```python
from build123d import *

# Parameters (mm, degrees)
F0_W     = 1168.9519882202
F0_H     = 1194.2882537842
F1_DEPTH = 152.4
F2_T     = 25.4


with BuildPart() as f1:
    # F0 (on Top) → F1 (new body)
    with BuildSketch(Plane.XY):
        Rectangle(F0_W, F0_H)
    extrude(amount=F1_DEPTH)

    # F2
    f2_openings = [f1.faces().sort_by_distance(p)[0] for p in [
        (0, 0, 0),
        (0, 0, 152.4),
    ]]
    offset(amount=F2_T, openings=f2_openings, kind=Kind.INTERSECTION)


solid = f1.part
```
CAD build for the part. Positions are in the model's coordinates, mm. A direction names the side the tool comes from. Give positions to 0.01 mm unless a question says otherwise; leave off trailing zeros. Loops run counter-clockwise (first coordinate to the right, second up) from the corner with the lowest first, then second, coordinate; pieces in that order, holes last. Notation, with made-up numbers: (-13.5, 76) -> (28.5, 76) arc R27 cw to (28.5, 101) -> close; hole circle Ø3 at (20, 35). An arc over 180 degrees is marked (long way). Use a Markdown table: item, result.
1. Mould opens along Y. For faces 1 (the flat face through (-8, -597.144, 75)), 2 (the flat face through (-590, 280, 152.4)), 3 (the flat face through (-584.476, -8, 75)), 4 (the flat face through (-9, 622.544, 75)) say: pulls with the +Y half, pulls with the -Y half, needs draft (parallel to the pull), parting line crosses it, or undercut.
Check result:
| item | result |
|---|---|
| face 1 | undercut |
| face 2 | needs draft |
| face 3 | undercut |
| face 4 | pulls with the +Y half |
2. Which spindle directions (+Z, -Z, +X, -X, +Y, -Y) get a long thin tool onto all of the face, cutting with end or side? Do faces 5 (the flat face through (-8, 597.144, 75)), 6 (the flat face through (-9, -622.544, 75)). Say none if no direction does.
Check result:
| item | result |
|---|---|
| face 5 | +Z, -Z |
| face 6 | +Z, -Z, +X, -X, -Y |
3. Wall check: L1, parallel to Y at x = -466, z = 145; L2, parallel to X at y = 194, z = 125. Give the ranges that are in metal, low to high. Write a range as [from, to].
Check result:
| item | result |
|---|---|
| L1 | y = [-622.54, -597.14], [597.14, 622.54] |
| L2 | x = [-609.88, -584.48], [584.48, 609.88] |
4. Slice it at C-C (z = 116.5). List the corners of the cut face in (x, y), plus the area to 3 significant figures.
Check result:
| item | result |
|---|---|
| outline | (-609.88, -622.54) -> (609.88, -622.54) -> (609.88, 622.54) -> (-609.88, 622.54) -> close; hole (-584.48, -597.14) -> (584.48, -597.14) -> (584.48, 597.14) -> (-584.48, 597.14) -> close |
| area | 123,000 mm^2 |
5. Slice it at B-B (x = -322.5). List the corners of the cut face in (y, z).
Check result:
| item | result |
|---|---|
| outline | (-622.54, 0) -> (-597.14, 0) -> (-597.14, 152.4) -> (-622.54, 152.4) -> close; (597.14, 0) -> (622.54, 0) -> (622.54, 152.4) -> (597.14, 152.4) -> close |
6. Slice it at A-A (y = -344). List the corners of the cut face in (x, z), plus the area to 3 significant figures.
Check result:
| item | result |
|---|---|
| outline | (-609.88, 0) -> (-584.48, 0) -> (-584.48, 152.4) -> (-609.88, 152.4) -> close; (584.48, 0) -> (609.88, 0) -> (609.88, 152.4) -> (584.48, 152.4) -> close |
| area | 7,740 mm^2 |
